Autodesk Inventor part; units mm, degrees
ref_plane "Work Plane2" through (-28.4982, 16.9145, 3.175) normal (1, 0, 0) x (0, 0, -1)
ref_plane "YZ Plane" through (0, 0, 0) normal (1, 0, 0) x (0, 1, 0)
ref_plane "XZ Plane" through (0, 0, 0) normal (0, 1, 0) x (-1, 0, 0)
sketch "Sketch1" plane through (0, 0, 0) normal (0, 0, 1) x (1, 0, 0)
  line L0 (-56.9976, 63.5) -> (0, 63.5)
  line L1 (0, 63.5) -> (-7.493, 63.5)
  line L2 (-7.493, 63.5) -> (-7.493, 57.15)
  line L3 (-56.9976, 63.5) -> (-49.5046, 63.5)
  line L4 (-49.5046, 63.5) -> (-49.5046, 57.15)
  line L5 (-56.9976, 63.5) -> (-56.9976, 0)
  line L6 (-56.9976, 0) -> (0, 0)
  line L7 (0, 0) -> (0, 63.5)
  line L8 (-28.4988, 0) -> (-28.4988, 11.1125)
  circle A0 centre (-28.4988, 11.1125) radius 4.7625
  dimension "d3" = 7.493
  dimension "d4" = 6.35
  dimension "d5" = 7.493
  dimension "d19" = 6.35
  dimension "d60" = 63.5
  dimension "d61" = 11.1125
  dimension "d62" = 9.525
extrude "Plate6" add sketch "Sketch1" along normal blind 3.175
sketch "Sketch6" plane through (0, 0, 0) normal (0, 0, -1) x (-1, 0, 0)
  line L0 (56.9976, 63.5) -> (56.9976, 0)
  line L1 (28.4988, 11.1125) -> (27.3076, 11.1125)
  line L2 (28.4988, 11.1125) -> (29.6894, 11.1125)
  circle A0 centre (28.4988, 11.1125) radius 4.7625
  circle A1 centre (28.4988, 11.1125) radius 4.7625
  line L3 (27.3076, 11.1125) -> (29.6888, 11.1125)
  line L4 (29.6888, 11.1125) -> (29.6888, 15.7239)
  line L5 (29.6888, 15.7239) -> (27.3076, 15.7239)
  line L6 (27.3076, 15.7239) -> (27.3076, 11.1125)
  line L7 (27.3076, 15.7239) -> (27.3076, 16.9145)
  line L8 (27.3076, 16.9145) -> (29.6888, 16.9145)
  line L9 (29.6888, 16.9145) -> (29.6888, 15.7239)
  point P0 (27.2012, 15.6948)
  point P1 (30.5454, 15.4129)
  dimension "d82" = 1.1906
  dimension "d86" = 2.3813
  dimension "d87" = 1.1906
extrude "Cut1" cut sketch "Sketch6" against normal blind 3.175 contours L7 L8 L9 A0 | A0 L5
sketch "Sketch7" plane through (-56.9976, 0, 0) normal (-1, 0, 0) x (0, 0, 1)
  line L0 (3.175, 0) -> (3.175, 63.5)
  line L1 (0, 63.5) -> (3.175, 63.5)
  line L2 (0, 63.5) -> (0, 0)
  line L3 (0, 0) -> (3.175, 0)
extrude "Extrusion2" add sketch "Sketch7" along normal blind 52.1462
sketch "Sketch8" plane through (0, 0, 3.175) normal (0, 0, 1) x (1, 0, 0)
  line L0 (0, 0) -> (-109.1438, 0)
  line L1 (-109.1438, 0) -> (-109.1438, 63.5)
  line L2 (-109.1438, 63.5) -> (-109.1438, 34.925)
  line L3 (-109.1438, 34.925) -> (-56.9976, 34.925)
  line L4 (-56.9976, 34.925) -> (-56.9976, 0)
  circle A0 centre (-75.5412, 57.15) radius 3.3782
  circle A1 centre (-75.5412, 41.275) radius 3.3782
  dimension "d71" = 28.575
  dimension "d72" = 52.1462
sketch "Sketch9" plane through (0, 0, 0) normal (0, 0, -1) x (-1, 0, 0)
  circle A0 centre (49.4976, 57.2287) radius 3.3
  circle A1 centre (7.4976, 57.2287) radius 3.3
extrude "Cut3" cut sketch "Sketch9" against normal blind 3.175
extrude "Cut4" cut sketch "Sketch8" against normal blind 3.175 contours L0 L1 L3 L4
sketch "Sketch10" plane through (0, 0, 3.175) normal (0, 0, 1) x (1, 0, 0)
  circle A0 centre (-90.6002, 57.15) radius 3.3782
  circle A1 centre (-90.6002, 41.275) radius 3.3782
extrude "Cut5" cut sketch "Sketch10" against normal blind 3.175
fillet "Fillet1" radius 25.4 2 edges at (-56.9976, 0, 1.5875) (0, 0, 1.5875)
sketch "Sketch11" plane through (0, 0, 3.175) normal (0, 0, 1) x (1, 0, 0)
  circle A0 centre (-90.6002, 57.15) radius 3.3782
  circle A1 centre (-90.6002, 41.275) radius 3.3782
  arc A2 (-25.4, 0) -> (0, 25.4) centre (-25.4, 25.4) ccw
  line L0 (0, 63.5) -> (0, 25.4)
  line L1 (-109.1438, 63.5) -> (0, 63.5)
  line L2 (-109.1438, 34.925) -> (-109.1438, 63.5)
  line L3 (-109.1438, 34.925) -> (-56.9976, 34.925)
  line L4 (-56.9976, 34.925) -> (-56.9976, 25.4)
  arc A3 (-56.9976, 25.4) -> (-31.5976, 0) centre (-31.5976, 25.4) ccw
  line L5 (-25.4, 0) -> (-31.5976, 0)
  circle A4 centre (-49.4976, 57.2287) radius 3.3
  circle A5 centre (-7.4976, 57.2287) radius 3.3
  line L6 (-29.6888, 15.7239) -> (-29.6888, 16.9145)
  line L7 (-29.6888, 16.9145) -> (-27.3076, 16.9145)
  line L8 (-27.3076, 16.9145) -> (-27.3076, 15.7239)
  line L9 (-27.3076, 15.7239) -> (-27.3088, 15.7239)
  arc A6 (-29.6888, 15.7239) -> (-27.3088, 15.7239) centre (-28.4988, 11.1125) ccw
  point P0 (0, 0)
ref_plane "Work Plane2" through (-28.4982, 16.9145, 3.175) normal (1, 0, 0) x (0, 0, -1)
sketch "Sketch12" plane through (0, 0, 0) normal (0, 0, -1) x (-1, 0, 0)
  arc A0 (0, 25.4) -> (25.4, 0) centre (25.4, 25.4) ccw
  line L0 (0, 63.5) -> (109.1438, 63.5)
  line L1 (0, 25.4) -> (0, 63.5)
  line L2 (27.3076, 16.9145) -> (29.6888, 16.9145)
  circle A1 centre (7.4976, 57.2287) radius 3.3
  circle A2 centre (28.4982, 58.7375) radius 3.175
  circle A3 centre (28.4982, 39.6875) radius 3.175
  line L3 (19.05, 63.5) -> (19.05, 0.8066)
  point P0 (0, 0)
  dimension "d88" = 19.05
extrude "Cut6" cut sketch "Sketch12" against normal blind 3.175
equation "\"d67\" = Thickness"
equation "\"d75\" = Thickness"
equation "\"d77\" = Thickness"
equation "\"d79\" = Thickness"
equation "\"d89\" = Thickness"
equation "\"BendRadius\" = Thickness"
equation "\"BendReliefWidth\" = Thickness"
equation "\"BendReliefDepth\" = 0.5 * Thickness"
equation "\"CornerReliefSize\" = 4 * Thickness"
equation "\"MinimumRemnant\" = 2 * Thickness"
equation "\"TransitionRadius\" = BendRadius"
equation "\"JacobiRadiusSize\" = BendRadius"
equation "\"GapSize\" = Thickness"
equation "\"d8\" = BendRadius"
equation "\"d56\" = BendRadius"
equation "\"d63\" = BendRadius"
properties part number "M - arm mount" material "Steel"
Work out the finished part from the listing and answer in its coordinate system (mm). A direction names the side the tool comes from. Coordinates: 2 decimals unless noted, no trailing zeros. Order: outer loops, then holes, each group sorted by start corner. A loop starts at its lowest first (then second) coordinate and runs counter-clockwise, first axis right, second up. Notation, with made-up numbers: M 85.5,75 L 100.5,75 A31 cw 100.5,100 Z; hole C 75,5.5 d8. An arc over 180 degrees is marked long. Use CSV: the item, a comma, the result in double quotes.
1) Flat-ended cylindrical pins translate along their axes: pin 1 Ø8.5 at (x, y) = (-28.5, 11.11) entering from -Z; pin 2 Ø1 at (x, z) = (-85, 1) entering from -Y (3 decimals); pin 3 Ø1.6 at (y, z) = (31.5, 1.5) entering from -X. Find the tip coordinate at first contact, or state that the pin passes through.
Worked out:
pin 1,"passes through"
pin 2,"stops at y = 34.925"
pin 3,"stops at x = -57"
2) For faces 5 (the face through (-83, 34.925, 2)), 6 (the face through (-28, 16.914, 2)), 7 (the face through (-109.144, 49, 2)), determine the directions among +Z, -Z, +X, -X, +Y, -Y from which every point of the face is accessible in a straight line to the end or side of a thin tool.
Worked out:
face 5,"+Z, -Z, -X, -Y"
face 6,"+Z, -Z"
face 7,"+Z, -Z, -X, +Y, -Y"
3) Consider line 1 (X direction, y = 60, z = 1.9) (3 decimals); line 2 (X direction, y = 56, z = 0.55); line 3 (X direction, y = 38.5, z = 2.35). Determine where each line is inside the solid, lowest interval first. Write a range as [from, to].
Worked out:
line 1,"x = [-109.144, -92.414], [-88.786, -51.289], [-47.706, -31.411], [-25.585, -19.05]"
line 2,"x = [-109.14, -93.78], [-87.42, -52.56], [-46.43, -30.11], [-26.89, -19.05]"
line 3,"x = [-109.14, -92.53], [-88.67, -31.44], [-25.55, -19.05]"
4) Determine the mould class of faces 1 (the face through (-88.784, 59.999, 1.61)), 2 (the face through (-28, 0, 2)), 3 (the face through (-28.085, 61.885, 1.565)), 4 (the face through (-22.244, 0.197, 1.61)) for opening direction X: released by +X, released by -X, zero draft, split by the parting line, or undercut.
Worked out:
face 1,"undercut"
face 2,"zero draft"
face 3,"undercut"
face 4,"released by +X"
5) Section B-B on z = 2.45 is taken. Count the separate pieces of the cut face and the enclosed holes in it, plus the area to 3 significant figures.
Worked out:
separate pieces,"1"
enclosed holes,"6"
area,"3,520 mm^2"
6) Section A-A on x = -91 is taken. Write down the section's boundary in (y, z) (3 decimals).
Worked out:
outline,"M 34.925,0 L 37.921,0 L 37.921,3.175 L 34.925,3.175 Z; M 44.629,0 L 53.796,0 L 53.796,3.175 L 44.629,3.175 Z; M 60.504,0 L 63.5,0 L 63.5,3.175 L 60.504,3.175 Z"
